Can you work these out from the drawing? Everything is in mm from the part's minimum corner. A direction names the side the tool comes from. Round coordinates to 2 decimals unless told otherwise and drop trailing zeros. Order: outer loops, then holes, each group sorted by start corner. A loop starts at its lowest first (then second) coordinate and runs counter-clockwise, first axis right, second up. Notation, with made-up numbers: M -7.75,75.25 L 39.25,75.25 A13 ccw 39.25,79.25 Z; hole C 65.5,74.25 d7. An arc over 180 degrees is marked long. Use one line per item in the form item = value. Start each with the question number.
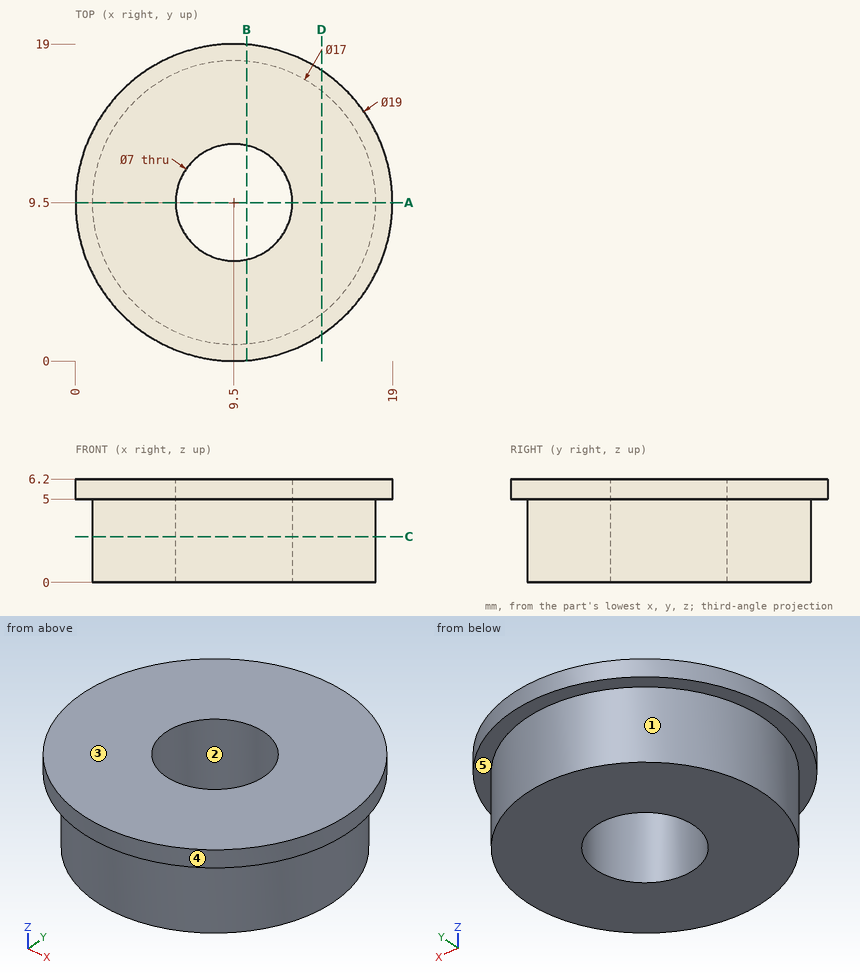
1) On a 3-axis mill with a long thin cutter (end or side, diameter ignored), from which of +Z, -Z, +X, -X, +Y, -Y can I reach the whole of each face in a straight line? I mean the marked faces 4 and 5. Say none if no direction works.
2) If we section it at B-B on x = 10.25: Write out the boundary of the cut face in (y, z), then the cut area to 3 significant figures.
3) If we mould it in two halves opening along Y, with no side actions, what happens to the marked faces 1, 2 and 3? For each: +Y half, -Y half, draft (parallel to the pull), parting line (faces both ways), or undercut.
4) Will these pins go through, and if not, where does the flat tip stop? pin 1 Ø6.5 at (x, y) = (9.5, 9.5) entering from +Z; pin 2 Ø3 at (x, y) = (14, 4) entering from -Z; pin 3 Ø1.5 at (x, z) = (14, 2.5) entering from -Y; pin 4 Ø2 at (x, z) = (12.5, 5) entering from +Y.
5) If I drill on line 1 (Y direction, x = 9.5, z = 4.5); line 2 (Y direction, x = 6.5, z = 1.75); line 3 (Z direction, x = 1, y = 11.75), over which ranges is the centre line in solid material (lowest first)?
6) If we section it at C-C on z = 2.75: Write out the boundary of the cut face in (x, y), then the cut area to 3 significant figures.
7) If we section it at D-D on x = 14.75: Write out the boundary of the cut face in (y, z).
8) If we section it at A-A on y = 9.5: Write out the boundary of the cut face in (x, z).
Completed:
q1.face_4 = +Z, -Z
q1.face_5 = -Z
q2.outline = M 0.03,5 L 1.03,5 L 1.03,0 L 6.08,0 L 6.08,6.2 L 0.03,6.2 Z; M 12.92,0 L 17.97,0 L 17.97,5 L 18.97,5 L 18.97,6.2 L 12.92,6.2 Z
q2.area = 65.0 mm²
q3.face_1 = parting line
q3.face_2 = undercut
q3.face_3 = draft
q4.pin_1 = through
q4.pin_2 = 0
q4.pin_3 = 1.87
q4.pin_4 = 18.79
q5.line_1 = 1 to 6, 13 to 18
q5.line_2 = 1.55 to 7.7, 11.3 to 17.45
q5.line_3 = 5 to 6.2
q6.outline = C 9.5,9.5 d17; hole C 9.5,9.5 d7
q6.area = 188 mm²
q7.outline = M 1.58,5 L 2.82,5 L 2.82,0 L 16.18,0 L 16.18,5 L 17.42,5 L 17.42,6.2 L 1.58,6.2 Z
q8.outline = M 0,5 L 1,5 L 1,0 L 6,0 L 6,6.2 L 0,6.2 Z; M 13,0 L 18,0 L 18,5 L 19,5 L 19,6.2 L 13,6.2 Z
